Work out the finished part from the listing and answer in its coordinate system (mm). A direction names the side the tool comes from. Round coordinates to 2 decimals unless told otherwise and drop trailing zeros. Order: outer loops, then holes, each group sorted by start corner. A loop starts at its lowest first (then second) coordinate and runs counter-clockwise, first axis right, second up. Notation, with made-up numbers: (-34.75, 83) -> (5.25, 83) arc R30 cw to (5.25, 108) -> close; hole circle Ø7 at (-11.5, 28.5). An arc over 180 degrees is marked (long way). Use one line per item in the form item = value.
```python
from build123d import *

# Parameters (mm, degrees)
SCHIZZO1_R                   = 2
ESTRUSIONE_ESTRUSIONE1_DEPTH = 5
FORO_PER_VITE_M3_1_D         = 3.4
FORO_PER_VITE_M3_1_DEPTH     = 12.5
FORO_FILETTATO_M3_1_D        = 2.5
FORO_FILETTATO_M3_1_DEPTH    = 4.5
FORO_FILETTATO_M3_1_TIP      = 0.751075774


with BuildPart() as part:
    # Schizzo1 → Estrusione-Estrusione1 (new body)
    with BuildSketch(Plane.XY):
        with BuildLine():
            Line((0, 30), (0, 0))
            Line((0, 0), (12.5, 0))
            Line((12.5, 0), (12.5, 5.015640289))
            ThreePointArc((12.5, 5.015640289), (13, 21), (13.5, 5.015640289))
            Line((13.5, 5.015640289), (13.5, 0))
            Line((13.5, 0), (30, 0))
            Line((30, 0), (30, 30))
            Line((30, 30), (0, 30))
        make_face()
        with Locations((25, 17)):
            Circle(SCHIZZO1_R, mode=Mode.SUBTRACT)
        with Locations((17, 25)):
            Circle(SCHIZZO1_R, mode=Mode.SUBTRACT)
    extrude(amount=ESTRUSIONE_ESTRUSIONE1_DEPTH)

    # Foro per Vite M3-1
    with Locations(Plane.ZY):
        with Locations((2.5, 2.507820144)):
            Hole(FORO_PER_VITE_M3_1_D / 2, depth=FORO_PER_VITE_M3_1_DEPTH)

    # Foro filettato M3-1
    with Locations(Plane.ZY.offset(-13.5)):
        with Locations((2.5, 2.507820144)):
            Hole(FORO_FILETTATO_M3_1_D / 2, depth=FORO_FILETTATO_M3_1_DEPTH)
            with Locations((0, 0, -(FORO_FILETTATO_M3_1_DEPTH + FORO_FILETTATO_M3_1_TIP / 2))):  # 118° drill point
                Cone(0, FORO_FILETTATO_M3_1_D / 2, FORO_FILETTATO_M3_1_TIP, mode=Mode.SUBTRACT)


solid = part.part
```
Item 1: For faces 1 (the cylindrical face through (6.34, 3.02, 0.88)), 2 (the cylindrical face through (13, 21, 2)), determine the directions among +Z, -Z, +X, -X, +Y, -Y from which every point of the face is accessible in a straight line to the end or side of a thin tool.
Findings:
face_1 = -X
face_2 = +Z, -Z
Item 2: Consider line 1 along X through (y, z) = (13, 3.85); line 2 along Y through (x, z) = (16.6, 2.5); line 3 along X through (y, z) = (18.25, 2.4). Determine where each line is inside the solid, lowest interval first.
Findings:
line_1 = 0 to 5, 21 to 30
line_2 = 0 to 1.26, 3.76 to 5.86, 20.14 to 23.04, 26.96 to 30
line_3 = 0 to 6.96, 19.04 to 23.44, 26.56 to 30
Item 3: A flat-ended cylindrical pin translates along its axis: P1, Ø3, axis at x = 17, y = 25, coming from the +Z side. Find the tip coordinate at first contact, or state that the pin passes through.
Findings:
P1 = through
Item 4: The part is cut by section B-B, the plane x = 8. Give the vertices of the cut face in (y, z) (3 decimals).
Findings:
outline = (0, 0) -> (6.755, 0) -> (6.755, 5) -> (0, 5) -> close; (19.245, 0) -> (30, 0) -> (30, 5) -> (19.245, 5) -> close; hole circle Ø3.4 at (2.508, 2.5)
Item 5: The part is cut by section A-A, the plane y = 25. Give the vertices of the cut face in (x, z).
Findings:
outline = (0, 0) -> (15, 0) -> (15, 5) -> (0, 5) -> close; (19, 0) -> (30, 0) -> (30, 5) -> (19, 5) -> close
Item 6: Determine the mould class of faces 3 (the flat face through (13.5, 3, 1)), 4 (the flat face through (15, 22, 5)), 5 (the flat face through (30, 15, 2)), 6 (the flat face through (0, 15, 2)) for opening direction X: released by +X, released by -X, zero draft, split by the parting line, or undercut.
Findings:
face_3 = undercut
face_4 = zero draft
face_5 = released by +X
face_6 = released by -X
Item 7: The part is cut by section D-D, the plane y = 17. Give the vertices of the cut face in (x, z), and give its area (3 significant figures).
Findings:
outline = (0, 0) -> (6.07, 0) -> (6.07, 5) -> (0, 5) -> close; (19.93, 0) -> (23, 0) -> (23, 5) -> (19.93, 5) -> close; (27, 0) -> (30, 0) -> (30, 5) -> (27, 5) -> close
area = 60.7 mm^2
